Here's the drawing with two shaded views (mm, measured from the low corner). I have some questions. A direction names the side the tool comes from. Give positions to 0.01 mm unless a question says otherwise; leave off trailing zeros. Loops run counter-clockwise (first coordinate to the right, second up) from the corner with the lowest first, then second, coordinate; pieces in that order, holes last. Notation, with made-up numbers: (-4.5, -6) -> (31.5, -6) arc R16 cw to (31.5, -2) -> close; hole circle Ø2 at (71, -18.5). An arc over 180 degrees is marked (long way). Answer in a Markdown table with one row per item. Add a question column.
Item 1: If we section it at A-A (x = 44): Write out the boundary of the cut face in (y, z).
Item 2: If we section it at B-B (y = 36.5): Write out the boundary of the cut face in (x, z).
Item 3: We'd pull the mould along Z, two halves only. Please class the marked faces 3, 4 and 5: released by +Z, released by -Z, zero draft, split by the parting line, or undercut.
Item 4: If we section it at D-D (y = 63): Write out the boundary of the cut face in (x, z), then the cut area to 3 significant figures.
Item 5: For P1, Ø17.5, axis at x = 62, z = 56.5, coming from the -Y side; P2, Ø15.5, axis at x = 28.5, y = 65.5, coming from the +Z side; P3, Ø2, axis at x = 58.5, z = 192.5, coming from the -Y side, each with a flat end and sliding along its axis, tell me the tip position at first contact or that it passes through.
Item 6: Which directions (+Z, -Z, +X, -X, +Y, -Y) give clear straight access to the entire face, cutting with the end or side of a thin tool? Please do the marked faces 1 and 2.
Item 7: If I drill on line 1 (X direction, y = 25, z = 135); line 2 (Z direction, x = 4, y = 49); line 3 (Z direction, x = 30, y = 24), over which ranges is the centre line in solid material (lowest first)?
Item 8: If we section it at C-C (z = 112.5): Write out the boundary of the cut face in (x, y) (1 decimal), then the cut area to 3 significant figures.
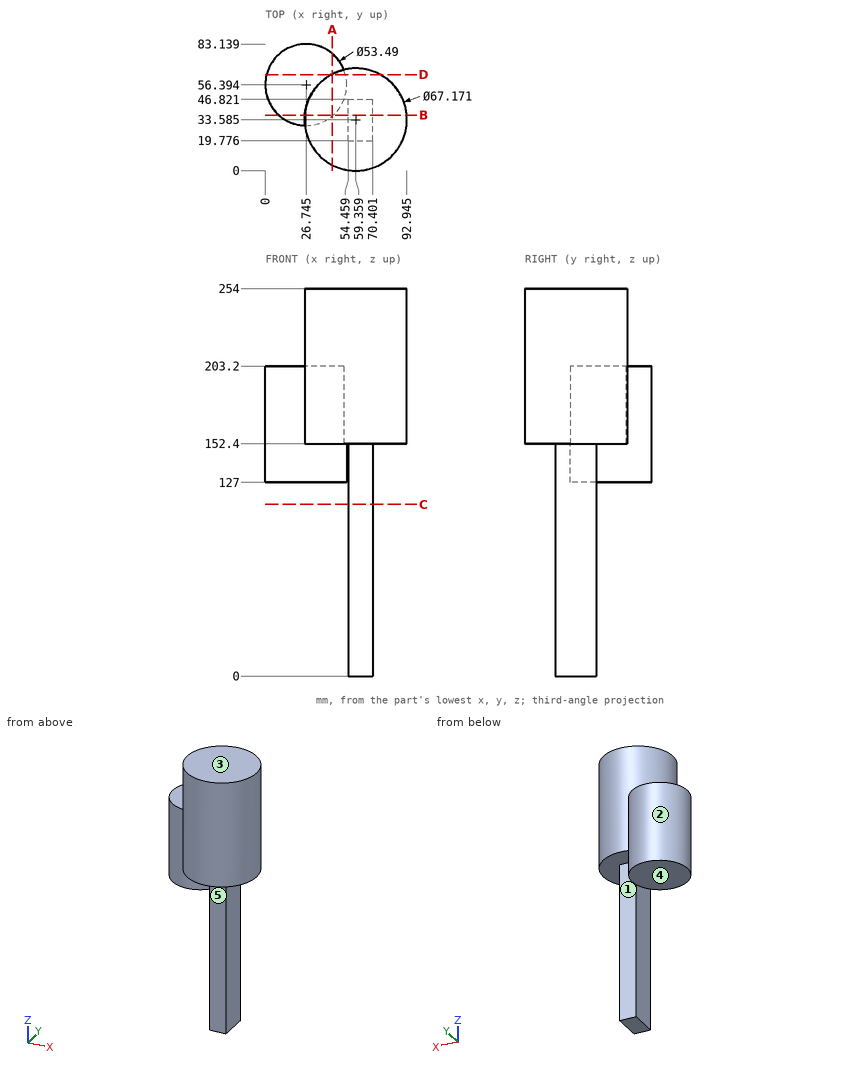
Recorded:
| question | item | result |
|---|---|---|
| 1 | outline | (3.72, 152.4) -> (35.96, 152.4) -> (35.96, 127) -> (76.83, 127) -> (76.83, 203.2) -> (63.45, 203.2) -> (63.45, 254) -> (3.72, 254) -> close |
| 2 | outline | (8.87, 127) -> (44.62, 127) -> (44.62, 152.4) -> (54.46, 152.4) -> (54.46, 0) -> (70.4, 0) -> (70.4, 152.4) -> (92.82, 152.4) -> (92.82, 254) -> (25.9, 254) -> (25.9, 203.2) -> (8.87, 203.2) -> close |
| 3 | face 3 | released by +Z |
| 3 | face 4 | released by -Z |
| 3 | face 5 | zero draft |
| 4 | outline | (0.83, 127) -> (52.66, 127) -> (52.66, 152.4) -> (75.57, 152.4) -> (75.57, 254) -> (43.15, 254) -> (43.15, 203.2) -> (0.83, 203.2) -> close |
| 4 | area | 6,760 mm^2 |
| 5 | P1 | stops at y = 19.78 |
| 5 | P2 | stops at z = 203.2 |
| 5 | P3 | stops at y = 0 |
| 6 | face 1 | -Z, +X, +Y |
| 6 | face 2 | -Z |
| 7 | line 1 | x = 54.46 to 70.4 |
| 7 | line 2 | z = 127 to 203.2 |
| 7 | line 3 | z = 152.4 to 254 |
| 8 | outline | (54.5, 19.8) -> (70.4, 19.8) -> (70.4, 46.8) -> (54.5, 46.8) -> close |
| 8 | area | 431 mm^2 |
